Autodesk Inventor part; units mm, degrees
ref_plane "YZ Plane" through (0, 0, 0) normal (1, 0, 0) x (0, 1, 0)
ref_plane "XZ Plane" through (0, 0, 0) normal (0, 1, 0) x (-1, 0, 0)
ref_plane "XY Plane" through (0, 0, 0) normal (0, 0, 1) x (1, 0, 0)
sketch "Sketch1" plane through (0, 0, 0) normal (0, 1, 0) x (-1, 0, 0)
  line L0 (-20, 10) -> (20, 10)
  line L1 (20, 10) -> (20, -10)
  line L2 (20, -10) -> (-20, -10)
  line L3 (-20, -10) -> (-20, 10)
  point P0 (0, 0)
  dimension "d0" = 40
  dimension "d1" = 20
  dimension "d2" = 10
  dimension "d3" = 20
extrude "Extrusion1" add sketch "Sketch1" along normal blind 1.6
sketch "Sketch2" plane through (0, 0, 0) normal (0, -1, 0) x (1, 0, 0)
  line L0 (20, 10) -> (-20, 10)
  line L1 (-20, 10) -> (-20, -10)
  line L2 (-20, -10) -> (20, -10)
  line L3 (20, -10) -> (20, 10)
  line L4 (-10, 0) -> (10, 0) construction
  line L5 (-10, -10) -> (10, -10)
  line L6 (10, 10) -> (-10, 10)
  arc A0 (-10, 10) -> (-10, -10) centre (-10, 0) ccw
  arc A1 (10, -10) -> (10, 10) centre (10, 0) ccw
  point P0 (0, 0)
  point P1 (0, 0)
  dimension "d6" = 10
extrude "Extrusion2" add sketch "Sketch2" along normal blind 1.6 contours A1 L2 A0 L0
sketch "Sketch3" plane through (0, -1.6, 0) normal (0, -1, 0) x (1, 0, 0)
  circle A0 centre (0, 0) radius 7.25
  dimension "d9" = 14.5
extrude "Extrusion3" add sketch "Sketch3" along normal blind 2.6
sketch "Sketch4" plane through (0, 1.6, 0) normal (0, 1, 0) x (1, 0, 0)
  line L0 (-18, -8) -> (18, -8) construction
  line L1 (18, -8) -> (18, 8) construction
  line L2 (18, 8) -> (-18, 8) construction
  line L3 (-18, 8) -> (-18, -8) construction
  line L4 (-18, -8) -> (18, 8) construction
  line L5 (18, -8) -> (-18, 8) construction
  point P0 (0, 0)
  dimension "d12" = 36
  dimension "d13" = 16
hole "Hole1" at (-18, 1.6, -8) at (-18, 1.6, 8) at (18, 1.6, 8) at (18, 1.6, -8) direction (0, -1, 0) diameter 2 end through all
properties part number "speaker"
Model file for the job. Use its own axes, mm. A direction names the side the tool comes from. Coordinates: 2 decimals unless noted, no trailing zeros. Loops run counter-clockwise (first coordinate to the right, second up) from the corner with the lowest first, then second, coordinate; pieces in that order, holes last. Notation, with made-up numbers: (-16.5, 89) - (40.5, 89) arc R15 ccw to (40.5, 100) - close; hole circle Ø6 at (39.5, -30). An arc over 180 degrees is marked (long way). Answer as a JSON object with one key per item and string values. Group by question number.
(1) Cut at C-C (x = -5). Give the cut face in (y, z), then the cut area to 3 significant figures.
(2) Cut at A-A (z = -8). Give the cut face in (x, y), then the cut area to 3 significant figures.
(3) Cut at B-B (x = -18). Give the cut face in (y, z).
(4) Tool access for faces 5 (the face through (16.9, 0, 7.6)), 6 (the face through (3.35, -2.88, 6.43)), 7 (the face through (-16.8, 0, 8)), 8 (the face through (-16.8, 0, -7.9)): list every direction of +Z, -Z, +X, -X, +Y, -Y with a clear straight run to the whole face (end or side of a thin tool).
(5) Two-plate mould, pull along X, no slides. Class faces 1 (the face through (19, 1, -8)), 2 (the face through (-20, -1, 0)), 3 (the face through (16.9, 0, -7.6)), 4 (the face through (20, -1, 0)): released by +X, released by -X, zero draft, split by the parting line, or undercut.
(6) Flat gauge pins, fed straight in: pin 1 (2.5 mm diameter, centred on x = 18, z = -8, fed in from -Y); pin 2 (4 mm diameter, centred on x = 14, z = -5.5, fed in from -Y). Where does each tip first touch, or does it go through?
(7) Probe line 1 along X through (y, z) = (0.9, -8); line 2 along Z through (x, y) = (18, 1.3); line 3 along Y through (x, z) = (-3.5, -7). List the from-to ranges inside material, lowest first.
(8) Cut at D-D (z = -4). Give the cut face in (x, y), then the cut area to 3 significant figures.
Geometry says:
{
 "1": {"outline": "(-4.2, -5.25) - (-1.6, -5.25) - (-1.6, -10) - (1.6, -10) - (1.6, 10) - (-1.6, 10) - (-1.6, 5.25) - (-4.2, 5.25) - close", "area": "91.3 mm^2"},
 "2": {"outline": "(-20, 0) - (-19, 0) - (-19, 1.6) - (-20, 1.6) - close; (-17, 0) - (-16, 0) - (-16, -1.6) - (16, -1.6) - (16, 0) - (17, 0) - (17, 1.6) - (-17, 1.6) - close; (19, 0) - (20, 0) - (20, 1.6) - (19, 1.6) - close", "area": "109 mm^2"},
 "3": {"outline": "(-1.6, -6) - (0, -6) - (0, -7) - (1.6, -7) - (1.6, 7) - (0, 7) - (0, 6) - (-1.6, 6) - close; (0, -10) - (1.6, -10) - (1.6, -9) - (0, -9) - close; (0, 9) - (1.6, 9) - (1.6, 10) - (0, 10) - close"},
 "4": {"face 5": "+Z, +X, -Y", "face 6": "-Y", "face 7": "+Z, -X, -Y", "face 8": "-Z, -X, -Y"},
 "5": {"face 1": "undercut", "face 2": "released by -X", "face 3": "zero draft", "face 4": "released by +X"},
 "6": {"pin 1": "stops at y = 0", "pin 2": "stops at y = -1.6"},
 "7": {"line 1": "x = -20 to -19, -17 to 17, 19 to 20", "line 2": "z = -10 to -9, -7 to 7, 9 to 10", "line 3": "y = -1.6 to 1.6"},
 "8": {"outline": "(-20, 0) - (-19.17, 0) - (-19.17, -1.6) - (-6.05, -1.6) - (-6.05, -4.2) - (6.05, -4.2) - (6.05, -1.6) - (19.17, -1.6) - (19.17, 0) - (20, 0) - (20, 1.6) - (-20, 1.6) - close", "area": "157 mm^2"}
}
